from build123d import *

# Parameters (mm, degrees)
SKETCH1_W           = 139.7
SKETCH1_H           = 439.61
BOSS_EXTRUDE1_DEPTH = 0.5
SKETCH2_W           = 139.7
SKETCH2_H           = 0.5
BOSS_EXTRUDE2_DEPTH = 12.7
FILLET1_R           = 1
FILLET2_R           = 1.5
SKETCH4_W           = 139.7
SKETCH4_H           = 0.5
BOSS_EXTRUDE3_DEPTH = 12.7
FILLET3_R           = 1
FILLET4_R           = 1.5


with BuildPart() as part:
    # Sketch1 → Boss-Extrude1 (new body)
    with BuildSketch(Plane(origin=(0, 0, 0), x_dir=(1, 0, 0), z_dir=(0, 1, 0))):
        with Locations((174.46911026, 72.328904153)):
            Rectangle(SKETCH1_W, SKETCH1_H)
    extrude(amount=BOSS_EXTRUDE1_DEPTH)

    # Sketch2 → Boss-Extrude2 (add)
    with BuildSketch(Plane.XZ):
        with Locations((174.46911026, 147.226095847)):
            Rectangle(SKETCH2_W, SKETCH2_H)
    extrude(amount=BOSS_EXTRUDE2_DEPTH)

    # Fillet1
    fillet1_edges = [part.edges().sort_by_distance(p)[0] for p in [
        (174.46911026, 0, 146.976095847),
    ]]
    fillet(fillet1_edges, radius=FILLET1_R)

    # Fillet2
    fillet2_edges = [part.edges().sort_by_distance(p)[0] for p in [
        (174.46911026, 0.5, 147.476095847),
    ]]
    fillet(fillet2_edges, radius=FILLET2_R)

    # Sketch4 → Boss-Extrude3 (add)
    with BuildSketch(Plane.XZ):
        with Locations((174.46911026, -291.883904153)):
            Rectangle(SKETCH4_W, SKETCH4_H)
    extrude(amount=BOSS_EXTRUDE3_DEPTH)

    # Fillet3
    fillet3_edges = [part.edges().sort_by_distance(p)[0] for p in [
        (174.46911026, 0, -291.633904153),
    ]]
    fillet(fillet3_edges, radius=FILLET3_R)

    # Fillet4
    fillet4_edges = [part.edges().sort_by_distance(p)[0] for p in [
        (174.46911026, 0.5, -292.133904153),
    ]]
    fillet(fillet4_edges, radius=FILLET4_R)


solid = part.part
Source: CAD feature listing. Evaluate the final solid. Frame: model axes, mm. A direction names the side the tool comes from. Round coordinates to 2 decimals unless told otherwise and drop trailing zeros. Order: outer loops, then holes, each group sorted by start corner. A loop starts at its lowest first (then second) coordinate and runs counter-clockwise, first axis right, second up. Notation, with made-up numbers: (79, 61.5) - (128, 61.5) arc R28 cw to (128, 90.5) - close; hole circle Ø5 at (-3, 25.5). An arc over 180 degrees is marked (long way). Use a Markdown table: item, result. Add a question column.
1. Line query: probe 1 along Z at (x, y) = (176, -12); probe 2 along Y at (x, z) = (230, 86.5). Output: solid intervals per line, ascending.
2. Section query A-A (y = -5). Return the cut outline in (x, z).
3. Section query C-C (z = 93). Return the cut outline in (x, y), then the cut area to 4 significant figures.
4. Set-up query: faces 5 (the flat face through (104.619, 0.3, -73.4)), 6 (the flat face through (173, 0, -75)). Return all of +Z, -Z, +X, -X, +Y, -Y with unobstructed straight access to the full face (end or side cutting, diameter ignored); none if empty.
5. Mould query, pull axis Z, two halves, no side actions, for faces 1 (the flat face through (244.319, 0.3, -73.4)), 2 (the flat face through (173, -7, -292.134)), 3 (the flat face through (173, -7, -291.634)), 4 (the flat face through (173, -7, 147.476)). Classes: +Z half, -Z half, draft (parallel to the pull), parting line (faces both ways), or undercut.
6. Section query B-B (x = 188.5). Return the cut outline in (y, z), then the cut area to 3 significant figures.
Derived:
| question | item | result |
|---|---|---|
| 1 | probe 1 | -292.13 to -291.63, 146.98 to 147.48 |
| 1 | probe 2 | 0 to 0.5 |
| 2 | outline | (104.62, -292.13) - (244.32, -292.13) - (244.32, -291.63) - (104.62, -291.63) - close; (104.62, 146.98) - (244.32, 146.98) - (244.32, 147.48) - (104.62, 147.48) - close |
| 3 | outline | (104.62, 0) - (244.32, 0) - (244.32, 0.5) - (104.62, 0.5) - close |
| 3 | area | 69.85 mm2 |
| 4 | face 5 | +Z, -Z, -X, +Y, -Y |
| 4 | face 6 | +X, -X, -Y |
| 5 | face 1 | draft |
| 5 | face 2 | -Z half |
| 5 | face 3 | undercut |
| 5 | face 4 | +Z half |
| 6 | outline | (-12.7, -292.13) - (-1, -292.13) arc R1.5 ccw to (0.5, -290.63) - (0.5, 145.98) arc R1.5 ccw to (-1, 147.48) - (-12.7, 147.48) - (-12.7, 146.98) - (-1, 146.98) arc R1 cw to (0, 145.98) - (0, -290.63) arc R1 cw to (-1, -291.63) - (-12.7, -291.63) - close |
| 6 | area | 232 mm2 |
